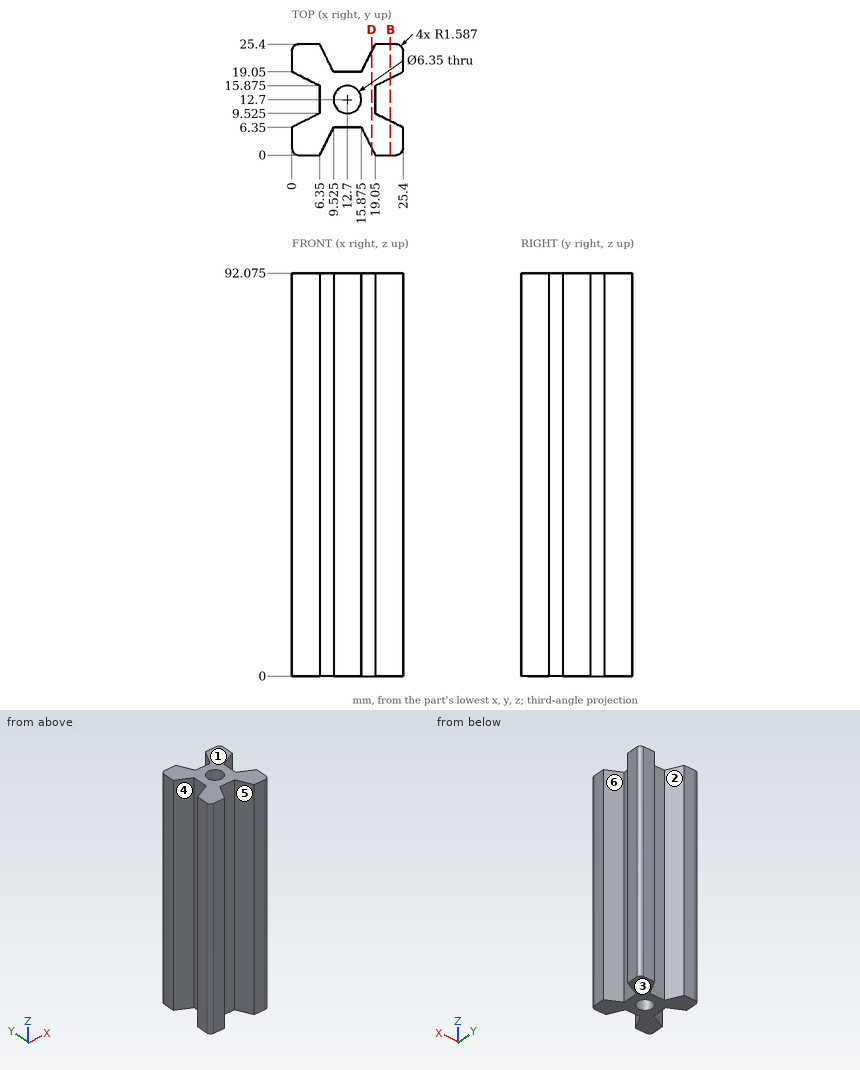
Drawing for the job (mm, zero at the part's lowest x, y, z). A direction names the side the tool comes from. Round coordinates to 2 decimals unless told otherwise and drop trailing zeros. Loops run counter-clockwise (first coordinate to the right, second up) from the corner with the lowest first, then second, coordinate; pieces in that order, holes last. Notation, with made-up numbers: M 73,-38.75 L 107,-38.75 A17 cw 107,-11.75 Z; hole C 79,-31 d10. An arc over 180 degrees is marked long. Use a Markdown table: item, result. Add a question column.
(1) Which spindle directions (+Z, -Z, +X, -X, +Y, -Y) get a long thin tool onto all of the face, cutting with end or side? Do the marked faces 1 and 2. Say none if no direction does.
(2) Cut at B-B (x = 22.5). Give the cut face in (y, z) (1 decimal), and give its area (3 significant figures).
(3) Pull direction X, two halves, no side cores. Call the marked faces 3, 4, 5 and 6: +X half, -X half, draft (parallel to the pull), parting line (faces both ways), or undercut.
(4) Flat gauge pins, fed straight in: pin 1 (1 mm diameter, centred on y = 13, z = 23.5, fed in from -X); pin 2 (1.9 mm diameter, centred on x = 14, z = 40.5, fed in from +Y); pin 3 (6 mm diameter, centred on y = 5.5, z = 41, fed in from -X); pin 4 (5 mm diameter, centred on y = 11.5, z = 32.5, fed in from -X). Where does each tip first touch, or does it go through?
(5) Drill centre lines: line 1 (X direction, y = 24.25, z = 13.5) (1 decimal); line 2 (Y direction, x = 11, z = 47); line 3 (Y direction, x = 20.5, z = 53.5). Where is each one in solid material? Low to high.
(6) Cut at D-D (x = 18.25). Give the cut face in (y, z) (1 decimal).
Geometry says:
| question | item | result |
|---|---|---|
| 1 | face 1 | +Z, +X, -X, +Y, -Y |
| 1 | face 2 | +Z, -Z, +Y |
| 2 | outline | M 0,0 L 7.8,0 L 7.8,92.1 L 0,92.1 Z; M 17.6,0 L 25.4,0 L 25.4,92.1 L 17.6,92.1 Z |
| 2 | area | 1,440 mm² |
| 3 | face 3 | draft |
| 3 | face 4 | -X half |
| 3 | face 5 | undercut |
| 3 | face 6 | +X half |
| 4 | pin 1 | stops at x = 6.35 |
| 4 | pin 2 | stops at y = 19.05 |
| 4 | pin 3 | stops at x = 0 |
| 4 | pin 4 | stops at x = 5.3 |
| 5 | line 1 | x = 0.1 to 6.9, 18.5 to 25.3 |
| 5 | line 2 | y = 6.35 to 10.02, 15.38 to 19.05 |
| 5 | line 3 | y = 0 to 8.8, 16.6 to 25.4 |
| 6 | outline | M 1.6,0 L 23.8,0 L 23.8,92.1 L 1.6,92.1 Z |
